Could you check a few things on this model? Use its own coordinates, in mm. Round coordinates to 2 decimals unless told otherwise and drop trailing zeros. Write each loop counter-clockwise with the first axis right and the second up, starting at its lowest first coordinate (ties: lowest second). Pieces come first, ordered by that corner, then holes. Notation, with made-up numbers: M -2,-32.75 L 37,-32.75 A22 cw 37,-6.75 Z; hole C 89.5,79 d9. An arc over 180 degrees is marked long. One line per item, written item: value. Start each with the question number.
(1) I want a section at C-C on y = -0.6. Please give me the cut outline in (x, z), and give its area (3 significant figures).
(2) If I drill on L1, parallel to Z at x = 0, y = -1.35; L2, parallel to Z at x = -0.95, y = -1.65; L3, parallel to Z at x = -2.15, y = -0.3, over which ranges is the centre line in solid material (lowest first)?
(3) Thinking about a two-plate mould opening in Z: for faces 1 (the face through (-2.5, -1, 1)), 2 (the face through (0, -1, -40)), 3 (the face through (0, -1, 36)), which applies, released by +Z, released by -Z, zero draft, split by the parting line, or undercut?
(4) I want a section at B-B on x = 0. Please give me the cut outline in (y, z).
(5) I want a section at A-A on z = 12.5. Please give me the cut outline in (x, y), and give its area (3 significant figures).
```python
from build123d import *

# Parameters (mm, degrees)
F0_R     = 1.5
F1_DEPTH = 2


with BuildPart() as f1:
    # F0 (on Front) → F1 (new body)
    with BuildSketch(Plane.XZ):
        with BuildLine():
            Line((2.5, -37.5), (2.5, 37.5))
            ThreePointArc((2.5, 37.5), (0, 40), (-2.5, 37.5))
            Line((-2.5, 37.5), (-2.5, -37.5))
            ThreePointArc((-2.5, -37.5), (0, -40), (2.5, -37.5))
        make_face()
        with Locations((0, -37.5)):
            Circle(F0_R, mode=Mode.SUBTRACT)
        with Locations((0, 12.5)):
            Circle(F0_R, mode=Mode.SUBTRACT)
        with Locations((0, 37.5)):
            Circle(F0_R, mode=Mode.SUBTRACT)
    extrude(amount=F1_DEPTH)


solid = f1.part
```
Found:
1. outline: M -2.5,-37.5 A2.5 ccw 2.5,-37.5 L 2.5,37.5 A2.5 ccw -2.5,37.5 Z; hole C 0,-37.5 d3; hole C 0,12.5 d3; hole C 0,37.5 d3
1. area: 373 mm²
2. L1: z = -40 to -39, -36 to 11, 14 to 36, 39 to 40
2. L2: z = -39.81 to -38.66, -36.34 to 11.34, 13.66 to 36.34, 38.66 to 39.81
2. L3: z = -38.78 to 38.78
3. face 1: zero draft
3. face 2: released by -Z
3. face 3: undercut
4. outline: M -2,-40 L 0,-40 L 0,-39 L -2,-39 Z; M -2,-36 L 0,-36 L 0,11 L -2,11 Z; M -2,14 L 0,14 L 0,36 L -2,36 Z; M -2,39 L 0,39 L 0,40 L -2,40 Z
5. outline: M -2.5,-2 L -1.5,-2 L -1.5,0 L -2.5,0 Z; M 1.5,-2 L 2.5,-2 L 2.5,0 L 1.5,0 Z
5. area: 4.00 mm²
